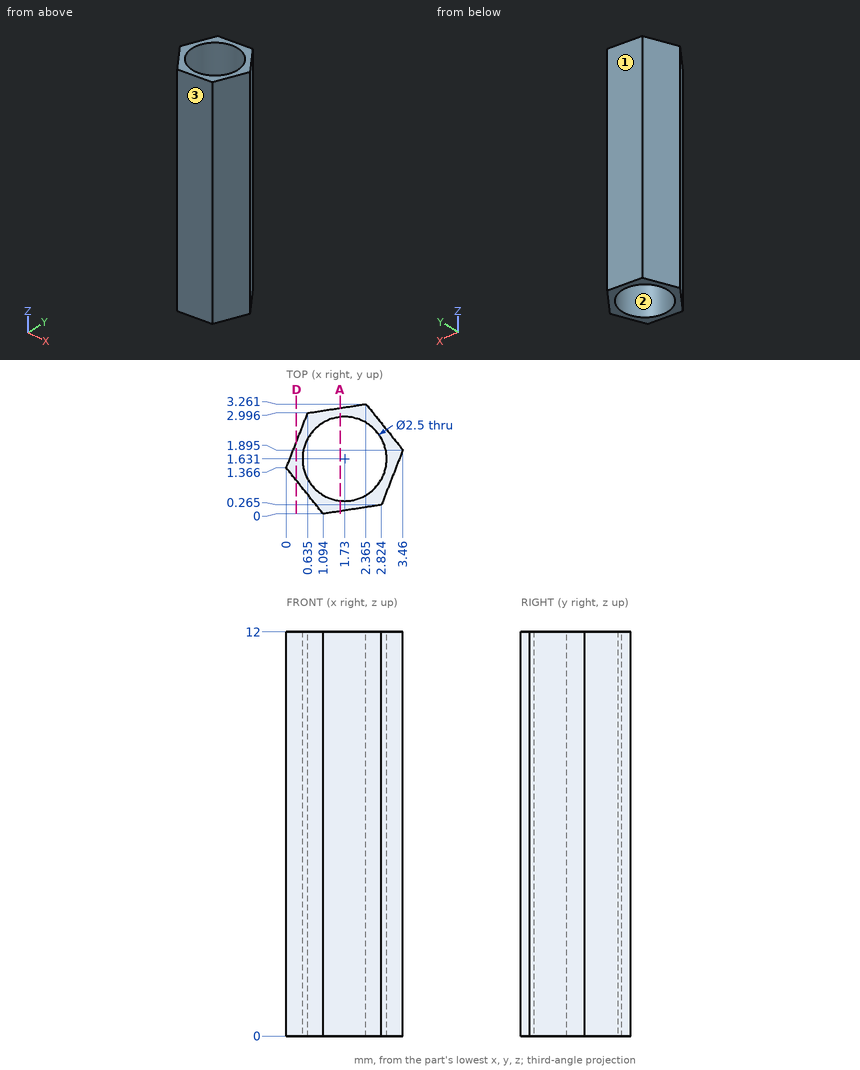
Job drawing, mm, ordinate dimensions from the low corner. One solid piece. Give positions to 0.01 mm unless a question says otherwise; leave off trailing zeros. Write each loop counter-clockwise with the first axis right and the second up, starting at its lowest first coordinate (ties: lowest second). Pieces come first, ordered by that corner, then holes. Notation, with made-up numbers: M 6.5,62.5 L 44.5,62.5 A28 ccw 44.5,88.5 Z; hole C 46,-9 d3. An arc over 180 degrees is marked long. One line per item, written item: value. Start each with the question number.
Q1. Saw through at A-A, the plane x = 1.6. Write the cut outline in (y, z).
Q2. Two-plate mould, pull along Y, no slides. Class the marked faces 1, 2 and 3: +Y half, -Y half, draft (parallel to the pull), parting line (faces both ways), or undercut.
Q3. Probe probe 1 along X at (y, z) = (1.4, 5) (1 decimal); probe 2 along X at (y, z) = (2.3, 4) (1 decimal); probe 3 along Y at (x, z) = (1.2, 11) (1 decimal). List the from-to ranges inside material, lowest first. Write a range as [from, to].
Q4. Saw through at D-D, the plane x = 0.3. Write the cut outline in (y, z) (1 decimal).
Q5. Drop flat-ended pins along their axis: pin 1 Ø1.5 at (x, z) = (0.5, 5) entering from -Y; pin 2 Ø1.5 at (y, z) = (1.5, 5.5) entering from +X. Give the stop position or say it passes through.
Output values:
1. outline: M 0.08,0 L 0.39,0 L 0.39,12 L 0.08,12 Z; M 2.87,0 L 3.14,0 L 3.14,12 L 2.87,12 Z
2. face 1: +Y half
2. face 2: undercut
2. face 3: -Y half
3. probe 1: x = [0, 0.5], [3, 3.3]
3. probe 2: x = [0.4, 0.7], [2.8, 3.1]
3. probe 3: y = [0, 0.5], [2.8, 3.1]
4. outline: M 1,0 L 2.1,0 L 2.1,12 L 1,12 Z
5. pin 1: stops at y = 0
5. pin 2: stops at x = 3.46
